from build123d import *

# Parameters (mm, degrees)
F0_W           = 43.6
F0_H           = 16.6
F1_DEPTH       = 1.5
F1_TAPER       = 20
F2_D           = 7
F2_CSINK_D     = 8
F2_CSINK_ANGLE = 90


with BuildPart() as f1:
    # F0 (on Top) → F1 (new body)
    with BuildSketch(Plane.XY):
        with Locations((-13.4155156434, -3.7059903711)):
            Rectangle(F0_W, F0_H)
    extrude(amount=F1_DEPTH, taper=F1_TAPER)

    # F2 (through all)
    with Locations(Plane(origin=(0, 0, 0), x_dir=(1, 0, 0), z_dir=(0, 0, -1))):
        with Locations((-27.5853313506, 4.0297852829), (-18.4464138001, 4.0297852829), (-8.8595086709, 4.0297852829), (0, 4.0297852829)):
            CounterSinkHole(F2_D / 2, F2_CSINK_D / 2, counter_sink_angle=F2_CSINK_ANGLE)


solid = f1.part
Work out the finished part from the listing and answer in its coordinate system (mm). Round coordinates to 2 decimals unless told otherwise and drop trailing zeros. Order: outer loops, then holes, each group sorted by start corner. A loop starts at its lowest first (then second) coordinate and runs counter-clockwise, first axis right, second up. Notation, with made-up numbers: M -32.5,-3 L 3.5,-3 A26 cw 3.5,14 Z; hole C 50,17.5 d1. An arc over 180 degrees is marked long. Put each result on its own line as item: value. Start each with the question number.
Q1. Section B-B, the plane z = 0.8 is taken. Write down the section's boundary in (x, y), and give its area (3 significant figures).
Q2. Section C-C, the plane y = -1 is taken. Give the number of separate pieces and of enclosed holes in the cut face, and give its area (3 significant figures).
Q3. Straight lines are drawn through the part: L1, parallel to X at y = -3.5, z = 1 (3 decimals); L2, parallel to X at y = -5, z = 0.8; L3, parallel to Y at x = -8, z = 0.95. For each, find the intervals that lie inside material, in ascending order. Write a range as [from, to].
Q4. For a pull along Y with two mould halves and no side action, classify faces 1 (the flat face through (-14, -4, 1.5)), 2 (the flat face through (-13.11, -11.737, 0.74)), 3 (the flat face through (-13.721, 4.325, 0.74)), 4 (the cylindrical face through (-14.95, -4.18, 1.01)) as pulls with the +Y half, pulls with the -Y half, needs draft (parallel to the pull), parting line crosses it, or undercut.
Q5. Flat-ended cylindrical pins translate along their axes: pin 1 (4 mm diameter, centred on x = -18.45, y = -4.03, fed in from +Z); pin 2 (1.5 mm diameter, centred on x = -4, y = -0.5, fed in from -Z). Find the tip coordinate at first contact, or state that the pin passes through.
Q6. Section A-A, the plane x = 0 is taken. Write down the section's boundary in (y, z), and give its area (3 significant figures).
Findings below:
1. outline: M -34.92,-11.71 L 8.09,-11.71 L 8.09,4.3 L -34.92,4.3 Z; hole C -27.59,-4.03 d7; hole C -18.45,-4.03 d7; hole C -8.86,-4.03 d7; hole C 0,-4.03 d7
1. area: 535 mm^2
2. separate pieces: 5
2. enclosed holes: 0
2. area: 41.8 mm^2
3. L1: x = [-34.852, -31.045], [-24.126, -21.906], [-14.987, -12.319], [-5.4, -3.46], [3.46, 8.021]
3. L2: x = [-34.92, -30.95], [-24.22, -21.81], [-15.08, -12.22], [-5.5, -3.36], [3.36, 8.09]
3. L3: y = [-11.66, -7.42], [-0.64, 4.25]
4. face 1: needs draft
4. face 2: pulls with the -Y half
4. face 3: pulls with the +Y half
4. face 4: undercut
5. pin 1: passes through
5. pin 2: stops at z = 0
6. outline: M -12.01,0 L -8.03,0 L -7.53,0.5 L -7.53,1.5 L -11.46,1.5 Z; M -0.53,0.5 L -0.03,0 L 4.59,0 L 4.05,1.5 L -0.53,1.5 Z
6. area: 13.3 mm^2
